Input: part model. Units: mm. Frame: model coordinates. Face numbers are marked on the shaded views. A direction names the side the tool comes from. Give positions to 0.01 mm unless a question says otherwise; leave off trailing zeros. Loops run counter-clockwise (first coordinate to the right, second up) from the corner with the lowest first, then second, coordinate; pieces in that order, holes last.
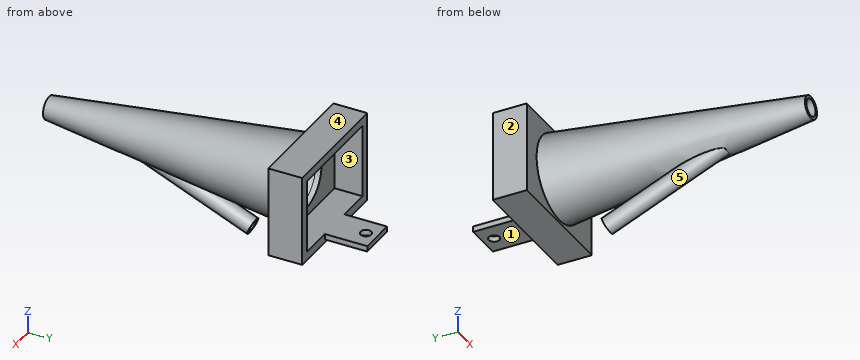
from build123d import *

# Parameters (mm, degrees)
SKETCH1_W           = 43
SKETCH1_H           = 32
SKETCH1_W_2         = 37
SKETCH1_H_2         = 26
BOSS_EXTRUDE1_DEPTH = 10
SKETCH2_W           = 13
SKETCH2_H           = 2
BOSS_EXTRUDE2_DEPTH = 15
CUT_EXTRUDE1_REACH  = 33
SKETCH3_R           = 1.905
SKETCH4_W           = 43
SKETCH4_H           = 32
BOSS_EXTRUDE3_DEPTH = 2
CUT_EXTRUDE2_REACH  = 29
SKETCH5_R           = 10
SKETCH14_R          = 3
BOSS_EXTRUDE4_DEPTH = 45
SKETCH16_R          = 2
CUT_EXTRUDE3_DEPTH  = 50


with BuildPart() as part:
    # Sketch1 → Boss-Extrude1 (new body)
    with BuildSketch(Plane(origin=(0, 0, 0), x_dir=(1, 0, 0), z_dir=(0, 1, 0))):
        with Locations((18.5, 13)):
            Rectangle(SKETCH1_W, SKETCH1_H)
        with Locations((18.5, 13)):
            Rectangle(SKETCH1_W_2, SKETCH1_H_2, mode=Mode.SUBTRACT)
    extrude(amount=BOSS_EXTRUDE1_DEPTH)

    # Sketch2 → Boss-Extrude2 (add)
    with BuildSketch(Plane(origin=(0, 10, 0), x_dir=(1, 0, 0), z_dir=(0, 1, 0))):
        with Locations((18.5, 27)):
            Rectangle(SKETCH2_W, SKETCH2_H)
    extrude(amount=BOSS_EXTRUDE2_DEPTH)

    # Sketch3 → Cut-Extrude1 (cut, up to next)
    with BuildSketch(Plane(origin=(0, 0, -28), x_dir=(-1, 0, 0), z_dir=(0, 0, -1)), mode=Mode.PRIVATE) as cut_extrude1_sk1:
        with Locations((-18.5, 21)):
            Circle(SKETCH3_R)
    cut_extrude1_tool1 = extrude(cut_extrude1_sk1.sketch, amount=-CUT_EXTRUDE1_REACH, mode=Mode.PRIVATE) & part.part
    add(cut_extrude1_tool1.solids().sort_by_distance((18.5, 21, -28))[0], mode=Mode.SUBTRACT)

    # Sketch4 → Boss-Extrude3 (add)
    with BuildSketch(Plane.XZ):
        with Locations((18.5, -13)):
            Rectangle(SKETCH4_W, SKETCH4_H)
    extrude(amount=BOSS_EXTRUDE3_DEPTH)

    # Sketch5 → Cut-Extrude2 (cut, up to next)
    with BuildSketch(Plane.XZ.offset(2), mode=Mode.PRIVATE) as cut_extrude2_sk1:
        with Locations((18.5, -13)):
            Circle(SKETCH5_R)
    cut_extrude2_tool1 = extrude(cut_extrude2_sk1.sketch, amount=-CUT_EXTRUDE2_REACH, mode=Mode.PRIVATE) & part.part
    add(cut_extrude2_tool1.solids().sort_by_distance((18.5, -2, -13))[0], mode=Mode.SUBTRACT)

    # Sketch9 → Revolve1 (revolve)
    with BuildSketch(Plane.XY.offset(-13)):
        Polygon((28.5, -2), (21.5, -90.9), (22.5, -90.9), (33.5, -2), align=None)
    revolve(axis=Axis((18.5, -2, -13), (0, -1, 0)))

    # Sketch14 → Boss-Extrude4 (add)
    with BuildSketch(Plane(origin=(18.5, -19.108562857, -35.499809934), x_dir=(-1, 0, 0), z_dir=(0, -0.922782119, 0.385322153))):
        with Locations((0.305660396, 0)):
            Circle(SKETCH14_R)
    extrude(amount=BOSS_EXTRUDE4_DEPTH)

    # Sketch16 → Cut-Extrude3 (cut)
    with BuildSketch(Plane(origin=(0, -3.648843771, 1.523631969), x_dir=(1, 0, 0), z_dir=(0, 0.922782119, -0.385322153))):
        with Locations((18.194339604, 40.1215424)):
            Circle(SKETCH16_R)
    extrude(amount=-CUT_EXTRUDE3_DEPTH, mode=Mode.SUBTRACT)


solid = part.part
(1) Cut plane B-B (x = 35). Return the cut outline in (y, z).
Values follow:
outline: (-2, -29) - (10, -29) - (10, -26) - (0, -26) - (0, 0) - (10, 0) - (10, 3) - (-2, 3) - close
(2) Ray query, probe 1 along Z at (x, y) = (26, 8); probe 2 along Z at (x, y) = (18.5, -1.1); probe 3 along Y at (x, z) = (11, -27.5). Return the intervals inside material, ascending.
Values follow:
probe 1: z = -29 to -26, 0 to 3
probe 2: z = -29 to -23, -3 to 3
probe 3: y = -2 to 10
(3) Mould query, pull axis Y, two halves, no side actions, for the marked faces 4 and 5. Classes: +Y half, -Y half, draft (parallel to the pull), parting line (faces both ways), or undercut.
Values follow:
face 4: draft
face 5: undercut
(4) Cut plane C-C (y = -5). Return the cut outline in (x, z).
Values follow:
outline: circle Ø29.26 at (18.5, -13); hole circle Ø19.53 at (18.5, -13)
(5) Cut plane D-D (y = -31). Count the separate pieces of the cut face and the enclosed holes in it, and give its area (3 significant figures).
Values follow:
separate pieces: 2
enclosed holes: 2
area: 239 mm2
(6) Reachability of the marked faces 1, 2 and 3 from +Z, -Z, +X, -X, +Y, -Y: full face, straight path, thin tool, end or side. Return the list, or none.
Values follow:
face 1: -Z, +X, -X, +Y
face 2: +Z, -Z, -X, +Y, -Y
face 3: +Y
(7) Cut plane A-A (y = 21). Return the cut outline in (x, z) (3 decimals).
Values follow:
outline: (12, -28) - (16.595, -28) - (16.595, -26) - (12, -26) - close; (20.405, -28) - (25, -28) - (25, -26) - (20.405, -26) - close
(8) Pin query (flat end, axial travel): pin 1 Ø12 at (x, y) = (12.5, 0) entering from -Z; pin 2 Ø2 at (y, z) = (15, -27) entering from -X; pin 3 Ø3 at (y, z) = (-51.5, -11.5) entering from -X (3 decimals). Return the tip coordinate at first contact, or that it passes through.
Values follow:
pin 1: stops at z = -29
pin 2: stops at x = 12
pin 3: stops at x = 9.495
